Verification items for the finished model (mm, model axes). A direction names the side the tool comes from. Coordinates: 2 decimals unless noted, no trailing zeros. Loops run counter-clockwise (first coordinate to the right, second up) from the corner with the lowest first, then second, coordinate; pieces in that order, holes last.
Q1. Access from +Z, -Z, +X, -X, +Y, -Y to the whole of each face (thin tool, end or side, straight path). Record for faces 3 (the face through (14.633, 0.028, 241.187)), 4 (the face through (1, 2, 123)).
Q2. Material ranges on probe 1 along Z at (x, y) = (-0.5, -1) (3 decimals); probe 2 along Z at (x, y) = (-17.5, 0.2), recorded low to high.
Q3. Mould release check, pull along X, two halves, no side actions. Record for faces 1 (the face through (-16.73, 0.03, 240.83)), 2 (the face through (-1, -2, 123)): +X half, -X half, draft (parallel to the pull), parting line (faces both ways), or undercut.
Q4. Go/stop test with a flat-tipped pin: P1, Ø1.5, axis at x = -12.5, y = 1.5, coming from the +Z side (3 decimals). Record where the tip stops, or that it passes through.
Q5. Sectioned sample at A-A (y = -1.1). Enter the section's corners in (x, z) (1 decimal), then the cut area to 3 significant figures.
Autodesk Inventor part; units mm, degrees
ref_plane "YZ Plane" through (0, 0, 0) normal (1, 0, 0) x (0, 1, 0)
ref_plane "XZ Plane" through (0, 0, 0) normal (0, 1, 0) x (-1, 0, 0)
ref_plane "XY Plane" through (0, 0, 0) normal (0, 0, 1) x (1, 0, 0)
sketch "Эскиз1" plane through (0, 0, 0) normal (0, 0, 1) x (1, 0, 0)
  line L0 (60, 2) -> (-60, 2)
  line L1 (-60, 2) -> (-60, -2)
  line L2 (-60, -2) -> (60, -2)
  line L3 (60, -2) -> (60, 2)
  line L4 (60, 2) -> (-60, -2) construction
  line L5 (-60, 2) -> (60, -2) construction
  point P0 (0, 0)
  dimension "d0" = 120
  dimension "d1" = 4
extrude "Выдавливание1" add sketch "Эскиз1" along normal blind 250
sketch "Эскиз2" plane through (-60, 2, 0) normal (0, 1, 0) x (1, 0, 0)
  line L0 (39.0177, -248.4604) -> (47.6438, -232.9811)
  line L1 (52.0114, -230.415) -> (65.6925, -230.415)
  line L2 (70.0601, -232.9811) -> (79.336, -249.6263)
  arc A0 (79.336, -249.6263) -> (79.5824, -250) centre (81.9565, -248.166) ccw
  arc A1 (36.3971, -250) -> (39.0177, -248.4604) centre (36.3971, -247) ccw
  arc A2 (70.0601, -232.9811) -> (65.6925, -230.415) centre (65.6925, -235.415) ccw
  arc A3 (52.0114, -230.415) -> (47.6438, -232.9811) centre (52.0114, -235.415) ccw
  line L3 (79.5824, -250) -> (36.3971, -250)
  line L4 (0, -250) -> (120, -250)
  line L5 (120, -250) -> (0, -250)
  point P0 (60, 0)
  point P1 (58.852, -247.058)
  point P2 (39.5541, -247.4978)
  point P3 (49.0738, -230.415)
  point P4 (68.6301, -230.415)
  point P5 (78.1498, -247.4978)
  point P6 (60, -250)
  point P7 (60, -250)
  dimension "d9" = 3
  dimension "d10" = 5
  dimension "d11" = 19.585
extrude "Выдавливание2" cut sketch "Эскиз2" against normal blind 4
properties part number "поперечная грань тела"
Geometry check:
1. face 3: +Z, +Y, -Y
1. face 4: +Z, -Z, +X, -X, +Y
2. probe 1: z = 0 to 230.415
2. probe 2: z = 0 to 242.21
3. face 1: undercut
3. face 2: draft
4. P1: stops at z = 234.585
5. outline: (-60, 0) - (60, 0) - (60, 250) - (19.6, 250) arc R3 ccw to (19.3, 249.6) - (10.1, 233) arc R5 cw to (5.7, 230.4) - (-8, 230.4) arc R5 cw to (-12.4, 233) - (-21, 248.5) arc R3 ccw to (-23.6, 250) - (-60, 250) - close
5. area: 29,400 mm2
